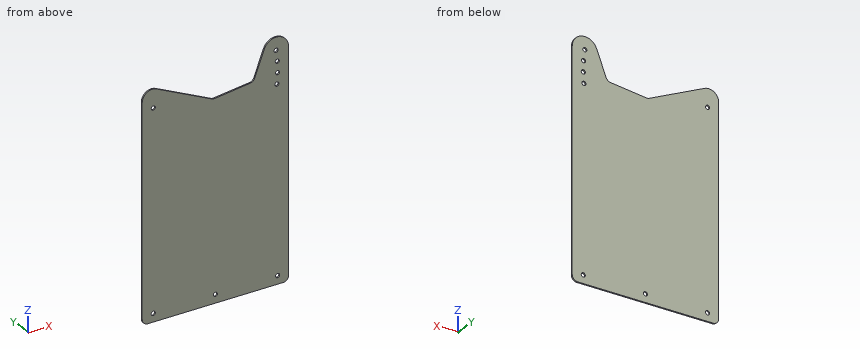
```python
from build123d import *

# Parameters (mm, degrees)
F1_R     = 4.7625
F2_DEPTH = 3.175
F3_R     = 12.7
F4_DEPTH = 50.8
F5_R     = 12.7
F6_R     = 4.7625
F7_DEPTH = 3.176


with BuildPart() as f2:
    # F1 (on Front) → F2 (new body)
    with BuildSketch(Plane.XZ):
        with BuildLine():
            Line((0, 438.0280625751), (0, 0))
            Line((0, 0), (336.55, 0))
            Line((336.55, 0), (336.55, 463.55))
            ThreePointArc((336.55, 463.55), (312.9733695253, 491.9375484372), (280.7399069367, 473.9732978163))
            Line((280.7399069367, 473.9732978163), (255.7973116004, 409.5266607723))
            Line((255.7973116004, 409.5266607723), (166.3505145476, 398.8620060081))
            Line((166.3505145476, 398.8620060081), (162.7768007124, 398.4359155775))
            Line((162.7768007124, 398.4359155775), (159.5108394321, 399.9480268652))
            Line((159.5108394321, 399.9480268652), (32.4645066839, 458.7693591847))
            ThreePointArc((32.4645066839, 458.7693591847), (10.5523855062, 457.2889027896), (0, 438.0280625751))
        make_face()
        with Locations((25.4, 419.1)):
            Circle(F1_R, mode=Mode.SUBTRACT)
        with Locations((309.5579415817, 388.9781352495)):
            Circle(F1_R, mode=Mode.SUBTRACT)
        with Locations((311.1019283196, 413.8587544951)):
            Circle(F1_R, mode=Mode.SUBTRACT)
        with Locations((310.4715508715, 438.7792627838)):
            Circle(F1_R, mode=Mode.SUBTRACT)
        with Locations((307.6716067903, 463.55)):
            Circle(F1_R, mode=Mode.SUBTRACT)
    extrude(amount=F2_DEPTH)

    # F3
    f3_edges = [f2.edges().sort_by_distance(p)[0] for p in [
        (162.776801, -1.5875, 398.435916),
        (255.797312, -1.5875, 409.526661),
    ]]
    fillet(f3_edges, radius=F3_R)

    # F4 (add): a face of the model
    f4_faces = [f2.faces().sort_by_distance(p)[0] for p in [
        (168.275, -1.5875, 0),
    ]]
    extrude(f4_faces, amount=F4_DEPTH)

    # F5
    f5_edges = [f2.edges().sort_by_distance(p)[0] for p in [
        (0, -1.5875, -50.8),
        (336.55, -1.5875, -50.8),
    ]]
    fillet(f5_edges, radius=F5_R)

    # F6 (on face) → F7 (cut, through all)
    with BuildSketch(Plane.XZ.offset(3.175)):
        with Locations((25.4, -31.75)):
            Circle(F6_R)
        with Locations((168.275, -31.75)):
            Circle(F6_R)
        with Locations((311.15, -31.75)):
            Circle(F6_R)
    extrude(amount=-F7_DEPTH, mode=Mode.SUBTRACT)


solid = f2.part
```
Geometry: final body of the model. Coordinates: model frame, mm. Give positions to 0.01 mm unless a question says otherwise; leave off trailing zeros. Order: outer loops, then holes, each group sorted by start corner. A loop starts at its lowest first (then second) coordinate and runs counter-clockwise, first axis right, second up. Notation, with made-up numbers: (68.5, 73) -> (101.5, 73) arc R23 cw to (101.5, 111) -> close; hole circle Ø9 at (68, 22.25). An arc over 180 degrees is marked (long way). Write each question's results on one line, items separated by ' | '. Start each with the question number.
1) Section B-B (x = 274.5). Return loops of the section in (y, z) (3 decimals), then the cut area to 3 significant figures.
2) Line query: line 1 (Z direction, x = 25.4, y = -0.95); line 2 (Z direction, x = 311.15, y = -1.5); line 3 (Z direction, x = 141, y = -1.2). Output: solid intervals per line, ascending. Write a range as from..to.
3) First-contact query: pin 1 (11 mm diameter, centred on x = 310.47, z = 438.78, fed in from -Y) (3 decimals); pin 2 (5.5 mm diameter, centred on x = 307.67, z = 463.55, fed in from +Y). Flat tips, straight axial feed; report the tip coordinate or a pass-through.
4) Section A-A (y = -1.9). Count the separate pieces of the cut face and the enclosed holes in it, then the cut area to 3 significant figures.
Calculated:
1) outline: (-3.175, -50.8) -> (0, -50.8) -> (0, 457.851) -> (-3.175, 457.851) -> close | area: 1,610 mm2
2) line 1: -50.8..-36.51, -26.99..414.34, 423.86..460.74 | line 2: -50.8..-36.51, -26.99..384.49, 393.47..409.1, 418.62..434.07, 443.49..460.3, 466.8..492.22 | line 3: -50.8..408.52
3) pin 1: y = -3.175 | pin 2: through
4) separate pieces: 1 | enclosed holes: 8 | area: 163,000 mm2
